from build123d import *

# Parameters (mm, degrees)
F0_R     = 6.35
F1_DEPTH = 4.826
F3_DEPTH = 24.13
F4_R     = 12.7
F5_R     = 12.7
F6_R     = 3.81
F7_DEPTH = 25.4


with BuildPart() as f1:
    # F0 (on Top) → F1 (new body)
    with BuildSketch(Plane.XY):
        with BuildLine():
            ThreePointArc((63.5, 11.43), (59.7802561211, 20.4102561211), (50.8, 24.13))
            Line((50.8, 24.13), (-63.5, 24.13))
            Line((-63.5, 24.13), (-63.5, -24.13))
            Line((-63.5, -24.13), (50.8, -24.13))
            ThreePointArc((50.8, -24.13), (59.7802561211, -20.4102561211), (63.5, -11.43))
            Line((63.5, -11.43), (63.5, 11.43))
        make_face()
        with Locations((-17.78, 0)):
            Circle(F0_R, mode=Mode.SUBTRACT)
        with BuildLine():
            Line((20.32, 6.35), (45.72, 6.35))
            ThreePointArc((45.72, 6.35), (52.07, 0), (45.72, -6.35))
            Line((45.72, -6.35), (20.32, -6.35))
            ThreePointArc((20.32, -6.35), (13.97, 0), (20.32, 6.35))
        make_face(mode=Mode.SUBTRACT)
    extrude(amount=F1_DEPTH)

    # F2 (on Front) → F3 (join, symmetric)
    with BuildSketch(Plane.XZ):
        with BuildLine():
            Line((-26.5013447812, 63.9799059919), (-71.4026253865, 19.0786253865))
            ThreePointArc((-71.4026253865, 19.0786253865), (-73.8252776553, 6.8991299599), (-63.5, 0))
            Line((-63.5, 0), (-63.5, 4.826))
            ThreePointArc((-63.5, 4.826), (-69.0200017902, 7.7421508405), (-69.7222982113, 13.9454673105))
            Line((-69.7222982113, 13.9454673105), (-23.2926998145, 60.3750657073))
            Line((-23.2926998145, 60.3750657073), (-26.5013447812, 63.9799059919))
        make_face()
    extrude(amount=F3_DEPTH, both=True)

    # F4
    f4_edges = [f1.edges().sort_by_distance(p)[0] for p in [
        (-24.897022, 24.13, 62.177486),
    ]]
    fillet(f4_edges, radius=F4_R)

    # F5
    f5_edges = [f1.edges().sort_by_distance(p)[0] for p in [
        (-24.897022, -24.13, 62.177486),
    ]]
    fillet(f5_edges, radius=F5_R)

    # F6 (on face) → F7 (cut)
    with BuildSketch(Plane(origin=(-45.2406253865, 0, 45.2406253865), x_dir=(0, -1, 0), z_dir=(-0.7071067812, 0, 0.7071067812))):
        with Locations((-12.7, 7.4513447812)):
            Circle(F6_R)
        with Locations((12.7, 7.4513447812)):
            Circle(F6_R)
    extrude(amount=-F7_DEPTH, mode=Mode.SUBTRACT)


solid = f1.part
Can you work these out from the model? Positions are in its coordinate system, mm. A direction names the side the tool comes from. Round coordinates to 2 decimals unless told otherwise and drop trailing zeros. Order: outer loops, then holes, each group sorted by start corner. A loop starts at its lowest first (then second) coordinate and runs counter-clockwise, first axis right, second up. Notation, with made-up numbers: (-7.75, 36) -> (47.25, 36) arc R10 cw to (47.25, 52) -> close; hole circle Ø6 at (20.5, 10). An arc over 180 degrees is marked (long way). Write each question's results on one line, items separated by ' | '. Start each with the question number.
Item 1: Thinking about a two-plate mould opening in Z: for faces 4 (the cylindrical face through (-40.92, -11.87, 46.2)), 5 (the flat face through (-1, 0, 4.826)), 6 (the cylindrical face through (52.07, 0.14, 2.38)), 7 (the cylindrical face through (-73.894, -0.338, 7.07)), which applies, +Z half, -Z half, draft (parallel to the pull), parting line (faces both ways), or undercut?
Item 2: Will these pins go through, and if not, where does the flat tip stop? pin 1 (1 mm diameter, centred on y = 4.5, z = 24.5, fed in from -X); pin 2 (1.5 mm diameter, centred on y = 0.5, z = 50, fed in from -X); pin 3 (14.5 mm diameter, centred on x = 3.5, y = 1, fed in from +Z); pin 4 (8 mm diameter, centred on y = 8, z = 10, fed in from -X).
Item 3: If we section it at B-B, the plane x = -17.78: Write out the boundary of the cut face in (y, z).
Item 4: If we section it at D-D, the plane x = 4.5: Write out the boundary of the cut face in (y, z).
Item 5: Please list where these lines run through material, in increasing order: L1, parallel to Z at x = 22.5, y = 18; L2, parallel to Z at x = -38.5, y = 15.5; L3, parallel to Z at x = -36, y = -19.
Item 6: Which directions (+Z, -Z, +X, -X, +Y, -Y) give clear straight access to the entire face, cutting with the end or side of a thin tool? Please do faces 1 (the flat face through (-48.64, -0.34, 41.84)), 2 (the flat face through (33, 6.35, 2)), 3 (the flat face through (-46.83, -0.34, 36.84)).
Item 7: If we section it at A-A, the plane y = 0: Write out the boundary of the cut face in (x, z) (1 decimal), then the cut area to 3 significant figures.
Item 8: If we section it at C-C, the plane y = 14: Write out the boundary of the cut face in (x, z) (1 decimal), then the cut area to 3 significant figures.
Results:
1) face 4: undercut | face 5: undercut | face 6: draft | face 7: parting line
2) pin 1: stops at x = -66.48 | pin 2: stops at x = -41.23 | pin 3: stops at z = 4.83 | pin 4: stops at x = -74.68
3) outline: (-24.13, 0) -> (-6.35, 0) -> (-6.35, 4.83) -> (-24.13, 4.83) -> close; (6.35, 0) -> (24.13, 0) -> (24.13, 4.83) -> (6.35, 4.83) -> close
4) outline: (-24.13, 0) -> (24.13, 0) -> (24.13, 4.83) -> (-24.13, 4.83) -> close
5) L1: z = 0 to 4.83 | L2: z = 0 to 4.83, 45.17 to 45.38 | L3: z = 0 to 4.83, 47.67 to 54.48
6) face 1: +Z, -X, +Y, -Y | face 2: +Z, -Z | face 3: +X, +Y, -Y
7) outline: (-71.4, 19.1) arc R11.2 ccw to (-63.5, 0) -> (-24.1, 0) -> (-24.1, 4.8) -> (-63.5, 4.8) arc R6.7 cw to (-69.7, 13.9) -> (-23.3, 60.4) -> (-26.5, 64) -> close; (-11.4, 0) -> (14, 0) -> (14, 4.8) -> (-11.4, 4.8) -> close; (52.1, 0) -> (63.5, 0) -> (63.5, 4.8) -> (52.1, 4.8) -> close | area: 770 mm2
8) outline: (-71.4, 19.1) arc R11.2 ccw to (-63.5, 0) -> (63.2, 0) -> (63.2, 4.8) -> (-63.5, 4.8) arc R6.7 cw to (-69.7, 13.9) -> (-39.1, 44.6) -> (-42.5, 48) -> close; (-37.4, 53) -> (-34, 49.6) -> (-23.5, 60.2) -> (-26.7, 63.8) -> close | area: 978 mm2
